Geometry check sheet. Reference: the model listing, model coordinates, mm. A direction names the side the tool comes from. Coordinates: 2 decimals unless noted, no trailing zeros. Write each loop counter-clockwise with the first axis right and the second up, starting at its lowest first coordinate (ties: lowest second). Pieces come first, ordered by that corner, then holes. Notation, with made-up numbers: M -17,23.25 L -6,23.25 A32 cw -6,50.25 Z; hole C -14,-35 d1. An arc over 180 degrees is marked long. Answer as a JSON object with one key per item and string values. Group by question number.
```python
from build123d import *

# Parameters (mm, degrees)
F2_SIZE = 1
F3_SIZE = 1.49999


# Not quite as in the source:
# - a fillet or chamfer is up to 0.001 mm smaller than in the source, because OpenCascade refuses the exact size


with BuildPart() as f1:
    # F0 (on Front) → F1 (revolve)
    with BuildSketch(Plane.XZ):
        Polygon((0, 8.5), (0, 3), (3.5, 3), (3.5, 10.75), (2, 10.75), (2, 8.5), align=None)
    revolve(axis=Axis((1.1402515594, 0, 0), (1, 0, 0)))

    # F2
    f2_edges = [f1.edges().sort_by_distance(p)[0] for p in [
        (3.5, 0, -3),
    ]]
    chamfer(f2_edges, length=F2_SIZE)

    # F3 (size 1.5 in the source; OpenCascade refuses exactly that, so slightly less here)
    f3_edges = [f1.edges().sort_by_distance(p)[0] for p in [
        (3.5, 0, -10.75),
    ]]
    chamfer(f3_edges, length=F3_SIZE)


solid = f1.part
```
1) Draft check along Z on faces 3 (the cylindrical face through (0.986, -7.167, 4.57)), 4 (the cylindrical face through (1, 0, -3)), 5 (the flat face through (0, 0, 4)). Enter one of: +Z half, -Z half, draft (parallel to the pull), parting line (faces both ways), or undercut.
2) Section check C-C (x = 0.55). Record the cut outline in (y, z), then the cut area to 3 significant figures.
3) Material ranges on probe 1 along Y at (x, z) = (1.8, 0); probe 2 along Z at (x, y) = (1.45, 7.5), recorded low to high. Write a range as [from, to].
4) Section check D-D (x = 3.25). Record the cut outline in (y, z), then the cut area to 3 significant figures.
5) Go/stop test with flat-tipped pins: pin 1 Ø5.5 at (y, z) = (0, 0) entering from -X; pin 2 Ø1.5 at (x, y) = (2, 4.5) entering from +Z; pin 3 Ø1.5 at (y, z) = (-7.5, -7.5) entering from -X. Record where each tip stops, or that it passes through.
6) Set-up check for faces 1 (the flat face through (2, -9, 1)), 2 (the flat face through (3.5, 4, -2)): record each of +Z, -Z, +X, -X, +Y, -Y from which the full face is reachable in a straight line by a thin tool's end or side.
Entries:
{
 "1": {"face 3": "parting line", "face 4": "undercut", "face 5": "draft"},
 "2": {"outline": "C 0,0 d17; hole C 0,0 d6", "area": "199 mm^2"},
 "3": {"probe 1": "[-8.5, -3], [3, 8.5]", "probe 2": "[-4, 4]"},
 "4": {"outline": "C 0,0 d19; hole C 0,0 d7.5", "area": "239 mm^2"},
 "5": {"pin 1": "through", "pin 2": "z = 10.07", "pin 3": "x = 2"},
 "6": {"face 1": "-X", "face 2": "+Z, -Z, +X, +Y, -Y"}
}
